```python
from build123d import *

# Parameters (mm, degrees)
SKETCH2_R                            = 40
BOSS_EXTRUDE1_DEPTH                  = 60
SKETCH3_R                            = 40
SKETCH3_R_2                          = 25
CUT_EXTRUDE1_DEPTH                   = 90
CHAMFER1_SIZE                        = 10
F_12_0_12_DIAMETER_HOLE1_D           = 12
F_12_0_12_DIAMETER_HOLE1_CSINK_D     = 12.05
F_12_0_12_DIAMETER_HOLE1_CSINK_ANGLE = 90


with BuildPart() as part:
    # Sketch2 → Boss-Extrude1 (new, symmetric)
    with BuildSketch(Plane.YZ):
        with Locations(Location((0, 0, 0), (0, 0, 90))):
            Circle(SKETCH2_R)
    extrude(amount=BOSS_EXTRUDE1_DEPTH, both=True)

    # Sketch3 → Cut-Extrude1 (cut)
    with BuildSketch(Plane.YZ.offset(60)):
        with Locations(Location((0, 0, 0), (0, 0, 90))):
            Circle(SKETCH3_R)
        with Locations(Location((0, 0, 0), (0, 0, 270))):
            Circle(SKETCH3_R_2, mode=Mode.SUBTRACT)
    extrude(amount=-CUT_EXTRUDE1_DEPTH, mode=Mode.SUBTRACT)

    # Chamfer1
    chamfer1_edges = [part.edges().sort_by_distance(p)[0] for p in [
        (-60, 0, -40),
        (60, 0, 25),
    ]]
    chamfer(chamfer1_edges, length=CHAMFER1_SIZE)

    # Ø12.0 (12) Diameter Hole1 (through all)
    with Locations(Plane(origin=(0, 25, 0), x_dir=(1, 0, 0), z_dir=(0, 1, 0))):
        with Locations((42, 0)):
            CounterSinkHole(F_12_0_12_DIAMETER_HOLE1_D / 2, F_12_0_12_DIAMETER_HOLE1_CSINK_D / 2, counter_sink_angle=F_12_0_12_DIAMETER_HOLE1_CSINK_ANGLE)


solid = part.part
```
The model under review builds one solid part; all positions refer to its coordinate system, in mm. A direction names the side the tool comes from. Coordinates: 2 decimals unless noted, no trailing zeros. Write each loop counter-clockwise with the first axis right and the second up, starting at its lowest first coordinate (ties: lowest second). Pieces come first, ordered by that corner, then holes.
1) We need section A-A on y = 0. State the section outline as (x, z) points.
2) We need section C-C on x = 10. State the section outline as (y, z) points, then the cut area to 3 significant figures.
3) We need section B-B on x = 38. State the section outline as (y, z) points, then the cut area to 3 significant figures.
4) Clearance check with flat-ended pins moving along their axes: pin 1 Ø5 at (y, z) = (1, 18) entering from +X; pin 2 Ø1 at (x, y) = (34, 8) entering from -Z; pin 3 Ø1 at (x, y) = (-24.5, 18.5) entering from -Z. State where each tip first meets the part, or that it passes through.
5) Machinability: for faces 5 (the face through (-60, 0, 0)), 6 (the face through (10.56, -24.406, 5.42)), which of the approach directions +Z, -Z, +X, -X, +Y, -Y give a long, thin tool a straight path to every point of the face, cutting with its end or side? Answer none if there is none.
6) The part is to be moulded in two halves that separate along X. For faces 1 (the face through (59.51, -15.12, 3.36)), 2 (the face through (48, 0, 0)), 3 (the face through (-59.514, 18.55, -24.192)), 4 (the face through (-39.86, 39.05, -8.67)), say which applies: pulls with the +X half, pulls with the -X half, needs draft (parallel to the pull), parting line crosses it, or undercut.
7) To check wall thickness, follow probe 1 along Z at (x, y) = (42, -6); probe 2 along Z at (x, y) = (42, 9); probe 3 along Z at (x, y) = (-2, 0.5) (3 decimals). State the ranges of each line that lie inside material, in increasing order.
8) We need section D-D on x = 52. State the section outline as (y, z) points, then the cut area to 3 significant figures.
Answer list:
1. outline: (-60, -30) - (-50, -40) - (-30, -40) - (-30, -25) - (50, -25) - (60, -15) - (60, 15) - (50, 25) - (-30, 25) - (-30, 40) - (-50, 40) - (-60, 30) - close; hole circle Ø12 at (42, 0)
2. outline: circle Ø50 at (0, 0)
2. area: 1,960 mm2
3. outline: (-24.6, -4.47) arc R25 ccw to (24.6, -4.47) - close; (-24.6, 4.47) - (24.6, 4.47) arc R25 ccw to start
3. area: 1,520 mm2
4. pin 1: stops at x = 59.47
4. pin 2: stops at z = -23.85
4. pin 3: stops at z = -17.35
5. face 5: +Z, -Z, -X, +Y, -Y
5. face 6: +X
6. face 1: pulls with the +X half
6. face 2: undercut
6. face 3: pulls with the -X half
6. face 4: needs draft
7. probe 1: z = -24.27 to -6, 6 to 24.27
7. probe 2: z = -23.32 to -6, 6 to 23.32
7. probe 3: z = -24.995 to 24.995
8. outline: circle Ø46 at (0, 0)
8. area: 1,660 mm2
